Design review of the part built by this model. Coordinates are the model's own, in mm. A direction names the side the tool comes from. Coordinates: 2 decimals unless noted, no trailing zeros. Loops run counter-clockwise (first coordinate to the right, second up) from the corner with the lowest first, then second, coordinate; pieces in that order, holes last. Notation, with made-up numbers: M 56,-2.75 L 99,-2.75 A8 ccw 99,10.25 Z; hole C 36,67 d4. An arc over 180 degrees is marked long. Answer as a JSON object with one key per item and string values. Group by question number.
1. Draft analysis for pull direction X (two halves, no side actions). For faces 1 (the cylindrical face through (0.087, 14.128, 2.93)), 2 (the cylindrical face through (128.24, -14.54, 3.01)), 3 (the flat face through (89, 31.344, 3)), state which applies: +X half, -X half, draft (parallel to the pull), parting line (faces both ways), or undercut.
2. Consider section B-B (x = 63.5). State the section outline as (y, z) points, then the cut area to 3 significant figures.
3. Insertion check: pin 1 (1.9 mm diameter, centred on x = 129.5, z = 4, fed in from -Y); pin 2 (1 mm diameter, centred on y = -17.5, z = 2, fed in from +X); pin 3 (3 mm diameter, centred on y = -2, z = 5, fed in from -X). Each pin has a flat end and moves straight along its axis. Give the tip position at first contact, or say it passes through.
4. Consider section A-A (x = 0). State the section outline as (y, z) points.
5. Machinability: for faces 4 (the flat face through (128.473, 22, 3)), 5 (the flat face through (-134, 25.4, 3)), 6 (the flat face through (-3.969, -2, 3)), 7 (the flat face through (113, 25.4, 3)), which of the approach directions +Z, -Z, +X, -X, +Y, -Y give a long, thin tool a straight path to every point of the face, cutting with its end or side? Answer none if there is none.
6. Consider section C-C (z = 1.5). Count the separate pieces of the cut face and the enclosed holes in it, then the cut area to 3 significant figures.
7. Consider section D-D (x = -29). State the section outline as (y, z) points, then the cut area to 3 significant figures.
8. To check wall thickness, follow probe 1 along X at (y, z) = (15.5, 2.7) (3 decimals); probe 2 along X at (y, z) = (18.5, 3.9); probe 3 along Y at (x, z) = (-63.5, 4.1). State the ranges of each line that lie inside material, in increasing order.
from build123d import *

# Parameters (mm, degrees)
BOSS_EXTRUDE1_DEPTH = 5.9436
CUT_EXTRUDE1_DEPTH  = 6.35
SKETCH3_R           = 4.826
CUT_EXTRUDE2_DEPTH  = 6.9436
CUT_EXTRUDE3_DEPTH  = 6.9436


with BuildPart() as part:
    # Sketch1 → Boss-Extrude1 (new body)
    with BuildSketch(Plane.XY):
        Polygon((-101.6, 25.4), (-101.6, 31.3436), (-76.2, 31.3436), (-76.2, 25.4), (76.2, 25.4), (76.2, 31.3436), (101.6, 31.3436), (101.6, 25.4), (139.7, 25.4), (139.7, -25.4), (-139.7, -25.4), (-139.7, 25.4), align=None)
    extrude(amount=BOSS_EXTRUDE1_DEPTH)

    # Sketch2 → Cut-Extrude1 (cut)
    with BuildSketch(Plane.XY.offset(5.9436)):
        Polygon((-128.4732, 25.4), (-128.4732, 17.62125), (-130.175, 17.62125), (-130.175, 15.24), (-128.4732, 15.24), (-128.4732, 12.7), (-125.5268, 12.7), (-125.5268, 15.24), (-123.825, 15.24), (-123.825, 17.62125), (-125.5268, 17.62125), (-125.5268, 25.4), align=None)
        Polygon((125.5268, 17.62125), (125.5268, 25.4), (128.4732, 25.4), (128.4732, 17.62125), (130.175, 17.62125), (130.175, 15.24), (128.4732, 15.24), (128.4732, 12.7), (125.5268, 12.7), (125.5268, 15.24), (123.825, 15.24), (123.825, 17.62125), align=None)
    extrude(amount=-CUT_EXTRUDE1_DEPTH, mode=Mode.SUBTRACT)

    # Sketch3 → Cut-Extrude2 (cut, through all)
    with BuildSketch(Plane(origin=(0, 0, 0), x_dir=(-1, 0, 0), z_dir=(0, 0, -1))):
        with Locations((-63.5, 5.9436)):
            Circle(SKETCH3_R)
        with Locations((63.5, 5.9436)):
            Circle(SKETCH3_R)
        with BuildLine():
            Line((3.96875, 10.16), (3.96875, -15.24))
            ThreePointArc((3.96875, -15.24), (0, -19.20875), (-3.96875, -15.24))
            Line((-3.96875, -15.24), (-3.96875, 10.16))
            ThreePointArc((-3.96875, 10.16), (0, 14.12875), (3.96875, 10.16))
        make_face()
    extrude(amount=-CUT_EXTRUDE2_DEPTH, mode=Mode.SUBTRACT)

    # Sketch4 → Cut-Extrude3 (cut, through all)
    with BuildSketch(Plane.XY.offset(5.9436)):
        with BuildLine():
            Line((-139.7, 12.7), (-139.7, -25.4))
            Line((-139.7, -25.4), (-101.6, -25.4))
            ThreePointArc((-101.6, -25.4), (-128.540768363, -14.240768363), (-139.7, 12.7))
        make_face()
        with BuildLine():
            Line((139.7, -25.4), (101.6, -25.4))
            ThreePointArc((101.6, -25.4), (128.540768363, -14.240768363), (139.7, 12.7))
            Line((139.7, 12.7), (139.7, -25.4))
        make_face()
    extrude(amount=-CUT_EXTRUDE3_DEPTH, mode=Mode.SUBTRACT)


solid = part.part
Findings below:
{
 "1": {"face 1": "undercut", "face 2": "+X half", "face 3": "draft"},
 "2": {"outline": "M -25.4,0 L 1.12,0 L 1.12,5.94 L -25.4,5.94 Z; M 10.77,0 L 25.4,0 L 25.4,5.94 L 10.77,5.94 Z", "area": "245 mm^2"},
 "3": {"pin 1": "stops at y = -14.23", "pin 2": "stops at x = 125.46", "pin 3": "stops at x = -137.34"},
 "4": {"outline": "M -25.4,0 L -19.21,0 L -19.21,5.94 L -25.4,5.94 Z; M 14.13,0 L 25.4,0 L 25.4,5.94 L 14.13,5.94 Z"},
 "5": {"face 4": "+Z, -Z, +Y", "face 5": "+Z, -Z, -X, +Y", "face 6": "+Z, -Z", "face 7": "+Z, -Z, +X, +Y"},
 "6": {"separate pieces": "1", "enclosed holes": "3", "area": "13,400 mm^2"},
 "7": {"outline": "M -25.4,0 L 25.4,0 L 25.4,5.94 L -25.4,5.94 Z", "area": "302 mm^2"},
 "8": {"probe 1": "x = -139.7 to -130.175, -123.825 to 123.825, 130.175 to 139.7", "probe 2": "x = -139.7 to -128.47, -125.53 to 125.53, 128.47 to 139.7", "probe 3": "y = -25.4 to 1.12, 10.77 to 25.4"}
}
